from build123d import *

# Parameters (mm, degrees)
F1_DEPTH = 25
F2_W     = 113.5
F2_H     = 53.5
F3_DEPTH = 5
F5_DEPTH = 133.9
F6_W     = 113.5
F6_H     = 60
F7_DEPTH = 5
F9_DEPTH = 25


with BuildPart() as f1:
    # F0 (on Front) → F1 (new body)
    with BuildSketch(Plane.XZ):
        with BuildLine():
            Line((30.7684078276, 51.75), (-82.7315921724, 51.75))
            Line((-82.7315921724, 51.75), (-82.7315921724, 37.7107225358))
            Line((-82.7315921724, 37.7107225358), (-77.4815921724, 37.7107225358))
            ThreePointArc((-77.4815921724, 37.7107225358), (-73.9815921724, 41.2107225358), (-70.4815921724, 37.7107225358))
            Line((-70.4815921724, 37.7107225358), (-65.4815921724, 37.7107225358))
            ThreePointArc((-65.4815921724, 37.7107225358), (-61.9815921724, 41.2107225358), (-58.4815921724, 37.7107225358))
            Line((-58.4815921724, 37.7107225358), (-54.4815921724, 37.7107225358))
            ThreePointArc((-54.4815921724, 37.7107225358), (-50.9815921724, 41.2107225358), (-47.4815921724, 37.7107225358))
            Line((-47.4815921724, 37.7107225358), (-42.4815921724, 37.7107225358))
            ThreePointArc((-42.4815921724, 37.7107225358), (-38.9815921724, 41.2107225358), (-35.4815921724, 37.7107225358))
            Line((-35.4815921724, 37.7107225358), (-30.4815921724, 37.7107225358))
            ThreePointArc((-30.4815921724, 37.7107225358), (-26.9815921724, 41.2107225358), (-23.4815921724, 37.7107225358))
            Line((-23.4815921724, 37.7107225358), (-18.4815921724, 37.7107225358))
            ThreePointArc((-18.4815921724, 37.7107225358), (-14.9815921724, 41.2107225358), (-11.4815921724, 37.7107225358))
            Line((-11.4815921724, 37.7107225358), (-6.4815921724, 37.7107225358))
            ThreePointArc((-6.4815921724, 37.7107225358), (-2.9815921724, 41.2107225358), (0.5184078276, 37.7107225358))
            Line((0.5184078276, 37.7107225358), (5.5184078276, 37.7107225358))
            ThreePointArc((5.5184078276, 37.7107225358), (9.0184078276, 41.2107225358), (12.5184078276, 37.7107225358))
            Line((12.5184078276, 37.7107225358), (17.5184078276, 37.7107225358))
            ThreePointArc((17.5184078276, 37.7107225358), (21.0184078276, 41.2107225358), (24.5184078276, 37.7107225358))
            Line((24.5184078276, 37.7107225358), (30.7684078276, 37.7107225358))
            Line((30.7684078276, 37.7107225358), (30.7684078276, 51.75))
        make_face()
        with BuildLine():
            Line((-77.4815921724, 12.7484267578), (-82.7315921724, 12.7484267578))
            Line((-82.7315921724, 12.7484267578), (-82.7315921724, -1.75))
            Line((-82.7315921724, -1.75), (30.7684078276, -1.75))
            Line((30.7684078276, -1.75), (30.7684078276, 12.7484267578))
            Line((30.7684078276, 12.7484267578), (25.5184078276, 12.7484267578))
            ThreePointArc((25.5184078276, 12.7484267578), (22.0184078276, 9.2484267578), (18.5184078276, 12.7484267578))
            Line((18.5184078276, 12.7484267578), (13.5184078276, 12.7484267578))
            ThreePointArc((13.5184078276, 12.7484267578), (10.0184078276, 9.2484267578), (6.5184078276, 12.7484267578))
            Line((6.5184078276, 12.7484267578), (1.5184078276, 12.7484267578))
            ThreePointArc((1.5184078276, 12.7484267578), (-1.9815921724, 9.2484267578), (-5.4815921724, 12.7484267578))
            Line((-5.4815921724, 12.7484267578), (-10.4815921724, 12.7484267578))
            ThreePointArc((-10.4815921724, 12.7484267578), (-13.9815921724, 9.2484267578), (-17.4815921724, 12.7484267578))
            Line((-17.4815921724, 12.7484267578), (-22.4815921724, 12.7484267578))
            ThreePointArc((-22.4815921724, 12.7484267578), (-25.9815921724, 9.2484267578), (-29.4815921724, 12.7484267578))
            Line((-29.4815921724, 12.7484267578), (-34.4815921724, 12.7484267578))
            ThreePointArc((-34.4815921724, 12.7484267578), (-37.9815921724, 9.2484267578), (-41.4815921724, 12.7484267578))
            Line((-41.4815921724, 12.7484267578), (-46.4815921724, 12.7484267578))
            ThreePointArc((-46.4815921724, 12.7484267578), (-49.9815921724, 9.2484267578), (-53.4815921724, 12.7484267578))
            Line((-53.4815921724, 12.7484267578), (-58.4815921724, 12.7484267578))
            ThreePointArc((-58.4815921724, 12.7484267578), (-61.9815921724, 9.2484267578), (-65.4815921724, 12.7484267578))
            Line((-65.4815921724, 12.7484267578), (-70.4815921724, 12.7484267578))
            ThreePointArc((-70.4815921724, 12.7484267578), (-73.9815921724, 9.2484267578), (-77.4815921724, 12.7484267578))
        make_face()
        with BuildLine():
            Line((-77.4815921724, 37.7107225358), (-82.7315921724, 37.7107225358))
            Line((-82.7315921724, 37.7107225358), (-82.7315921724, 12.7484267578))
            Line((-82.7315921724, 12.7484267578), (-77.4815921724, 12.7484267578))
            ThreePointArc((-77.4815921724, 12.7484267578), (-73.9815921724, 16.2484267578), (-70.4815921724, 12.7484267578))
            Line((-70.4815921724, 12.7484267578), (-65.4815921724, 12.7484267578))
            ThreePointArc((-65.4815921724, 12.7484267578), (-61.9815921724, 16.2484267578), (-58.4815921724, 12.7484267578))
            Line((-58.4815921724, 12.7484267578), (-53.4815921724, 12.7484267578))
            ThreePointArc((-53.4815921724, 12.7484267578), (-49.9815921724, 16.2484267578), (-46.4815921724, 12.7484267578))
            Line((-46.4815921724, 12.7484267578), (-41.4815921724, 12.7484267578))
            ThreePointArc((-41.4815921724, 12.7484267578), (-37.9815921724, 16.2484267578), (-34.4815921724, 12.7484267578))
            Line((-34.4815921724, 12.7484267578), (-29.4815921724, 12.7484267578))
            ThreePointArc((-29.4815921724, 12.7484267578), (-25.9815921724, 16.2484267578), (-22.4815921724, 12.7484267578))
            Line((-22.4815921724, 12.7484267578), (-17.4815921724, 12.7484267578))
            ThreePointArc((-17.4815921724, 12.7484267578), (-13.9815921724, 16.2484267578), (-10.4815921724, 12.7484267578))
            Line((-10.4815921724, 12.7484267578), (-5.4815921724, 12.7484267578))
            ThreePointArc((-5.4815921724, 12.7484267578), (-1.9815921724, 16.2484267578), (1.5184078276, 12.7484267578))
            Line((1.5184078276, 12.7484267578), (6.5184078276, 12.7484267578))
            ThreePointArc((6.5184078276, 12.7484267578), (10.0184078276, 16.2484267578), (13.5184078276, 12.7484267578))
            Line((13.5184078276, 12.7484267578), (18.5184078276, 12.7484267578))
            ThreePointArc((18.5184078276, 12.7484267578), (22.0184078276, 16.2484267578), (25.5184078276, 12.7484267578))
            Line((25.5184078276, 12.7484267578), (30.7684078276, 12.7484267578))
            Line((30.7684078276, 12.7484267578), (30.7684078276, 37.7107225358))
            Line((30.7684078276, 37.7107225358), (24.5184078276, 37.7107225358))
            ThreePointArc((24.5184078276, 37.7107225358), (21.0184078276, 34.2107225358), (17.5184078276, 37.7107225358))
            Line((17.5184078276, 37.7107225358), (12.5184078276, 37.7107225358))
            ThreePointArc((12.5184078276, 37.7107225358), (9.0184078276, 34.2107225358), (5.5184078276, 37.7107225358))
            Line((5.5184078276, 37.7107225358), (0.5184078276, 37.7107225358))
            ThreePointArc((0.5184078276, 37.7107225358), (-2.9815921724, 34.2107225358), (-6.4815921724, 37.7107225358))
            Line((-6.4815921724, 37.7107225358), (-11.4815921724, 37.7107225358))
            ThreePointArc((-11.4815921724, 37.7107225358), (-14.9815921724, 34.2107225358), (-18.4815921724, 37.7107225358))
            Line((-18.4815921724, 37.7107225358), (-23.4815921724, 37.7107225358))
            ThreePointArc((-23.4815921724, 37.7107225358), (-26.9815921724, 34.2107225358), (-30.4815921724, 37.7107225358))
            Line((-30.4815921724, 37.7107225358), (-35.4815921724, 37.7107225358))
            ThreePointArc((-35.4815921724, 37.7107225358), (-38.9815921724, 34.2107225358), (-42.4815921724, 37.7107225358))
            Line((-42.4815921724, 37.7107225358), (-47.4815921724, 37.7107225358))
            ThreePointArc((-47.4815921724, 37.7107225358), (-50.9815921724, 34.2107225358), (-54.4815921724, 37.7107225358))
            Line((-54.4815921724, 37.7107225358), (-58.4815921724, 37.7107225358))
            ThreePointArc((-58.4815921724, 37.7107225358), (-61.9815921724, 34.2107225358), (-65.4815921724, 37.7107225358))
            Line((-65.4815921724, 37.7107225358), (-70.4815921724, 37.7107225358))
            ThreePointArc((-70.4815921724, 37.7107225358), (-73.9815921724, 34.2107225358), (-77.4815921724, 37.7107225358))
        make_face()
    extrude(amount=F1_DEPTH)

    # F2 (on face) → F3 (join)
    with BuildSketch(Plane(origin=(0, 0, 0), x_dir=(-1, 0, 0), z_dir=(0, 1, 0))):
        with Locations((25.9815921724, 25)):
            Rectangle(F2_W, F2_H)
    extrude(amount=F3_DEPTH)

    # F4 (on face) → F5 (cut)
    with BuildSketch(Plane(origin=(-82.7315921724, 0, 0), x_dir=(0, -1, 0), z_dir=(-1, 0, 0))):
        Polygon((25, -1.75), (25, 51.75), (16.1387622356, -1.75), align=None)
    extrude(amount=-F5_DEPTH, mode=Mode.SUBTRACT)

    # F6 (on face) → F7 (join)
    with BuildSketch(Plane.XY.offset(51.75)):
        with Locations((-25.9815921724, -25)):
            Rectangle(F6_W, F6_H)
    extrude(amount=F7_DEPTH)

    # F8 (on face) → F9 (cut)
    with BuildSketch(Plane(origin=(0, 0, 51.75), x_dir=(1, 0, 0), z_dir=(0, 0, -1))):
        with BuildLine():
            ThreePointArc((-63.7315921724, 45), (-65.9815921724, 47.25), (-68.2315921724, 45))
            Line((-68.2315921724, 45), (-63.7315921724, 45))
        make_face()
        with BuildLine():
            ThreePointArc((16.2684078276, 45), (14.0184078276, 47.25), (11.7684078276, 45))
            Line((11.7684078276, 45), (16.2684078276, 45))
        make_face()
        with BuildLine():
            Line((16.2684078276, 45), (11.7684078276, 45))
            ThreePointArc((11.7684078276, 45), (14.0184078276, 42.75), (16.2684078276, 45))
        make_face()
        with BuildLine():
            ThreePointArc((-23.7315921724, 45), (-25.9815921724, 47.25), (-28.2315921724, 45))
            Line((-28.2315921724, 45), (-23.7315921724, 45))
        make_face()
        with BuildLine():
            Line((-23.7315921724, 45), (-28.2315921724, 45))
            ThreePointArc((-28.2315921724, 45), (-25.9815921724, 42.75), (-23.7315921724, 45))
        make_face()
        with BuildLine():
            Line((-63.7315921724, 45), (-68.2315921724, 45))
            ThreePointArc((-68.2315921724, 45), (-65.9815921724, 42.75), (-63.7315921724, 45))
        make_face()
        with BuildLine():
            ThreePointArc((-63.7315921724, 35), (-65.9815921724, 37.25), (-68.2315921724, 35))
            Line((-68.2315921724, 35), (-63.7315921724, 35))
        make_face()
        with BuildLine():
            ThreePointArc((16.2684078276, 35), (14.0184078276, 37.25), (11.7684078276, 35))
            Line((11.7684078276, 35), (16.2684078276, 35))
        make_face()
        with BuildLine():
            Line((16.2684078276, 35), (11.7684078276, 35))
            ThreePointArc((11.7684078276, 35), (14.0184078276, 32.75), (16.2684078276, 35))
        make_face()
        with BuildLine():
            ThreePointArc((-23.7315921724, 35), (-25.9815921724, 37.25), (-28.2315921724, 35))
            Line((-28.2315921724, 35), (-23.7315921724, 35))
        make_face()
        with BuildLine():
            Line((-23.7315921724, 35), (-28.2315921724, 35))
            ThreePointArc((-28.2315921724, 35), (-25.9815921724, 32.75), (-23.7315921724, 35))
        make_face()
        with BuildLine():
            Line((-63.7315921724, 35), (-68.2315921724, 35))
            ThreePointArc((-68.2315921724, 35), (-65.9815921724, 32.75), (-63.7315921724, 35))
        make_face()
    extrude(amount=-F9_DEPTH, mode=Mode.SUBTRACT)


solid = f1.part
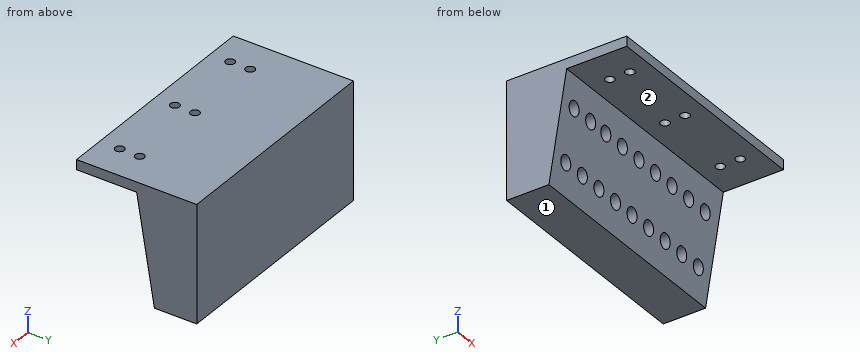
Source: CAD feature listing. Evaluate the final solid. Frame: model axes, mm. Face numbers are marked on the shaded views. A direction names the side the tool comes from. Give positions to 0.01 mm unless a question says otherwise; leave off trailing zeros. Order: outer loops, then holes, each group sorted by start corner. A loop starts at its lowest first (then second) coordinate and runs counter-clockwise, first axis right, second up. Notation, with made-up numbers: (46.25, 45) -> (81.25, 45) arc R20 cw to (81.25, 50) -> close; hole circle Ø8 at (-11.75, 57). An arc over 180 degrees is marked (long way). Use a Markdown table: item, result.
1) Section query B-B, the plane x = -32.5. Return the cut outline in (y, z), then the cut area to 3 significant figures.
Answer list:
| item | result |
|---|---|
| outline | (-55, 51.75) -> (-25, 51.75) -> (-16.14, -1.75) -> (5, -1.75) -> (5, 56.75) -> (-55, 56.75) -> close |
| area | 1,670 mm² |
2) Section query C-C, the plane y = -21. Count the separate pieces of the cut face and the enclosed holes in it, then the cut area to 3 significant figures.
Answer list:
| item | result |
|---|---|
| separate pieces | 1 |
| enclosed holes | 9 |
| area | 2,960 mm² |
3) Contact query for flat-ended pins moving along their axis: P1, Ø3, axis at x = -55, y = -38.5, coming from the -Z side; P2, Ø6.5, axis at x = -13.98, z = 12.75, coming from the -Y side; P3, Ø5, axis at x = -46.5, z = 20, coming from the -Y side. Output: stop coordinate, or through.
Answer list:
| item | result |
|---|---|
| P1 | z = 51.75 |
| P2 | y = 0 |
| P3 | y = -20.16 |
4) Section query A-A, the plane y = -45. Return the cut outline in (x, z), then the cut area to 3 significant figures.
Answer list:
| item | result |
|---|---|
| outline | (-82.73, 51.75) -> (-68.23, 51.75) -> (-68.23, 56.75) -> (-82.73, 56.75) -> close; (-63.73, 51.75) -> (-28.23, 51.75) -> (-28.23, 56.75) -> (-63.73, 56.75) -> close; (-23.73, 51.75) -> (11.77, 51.75) -> (11.77, 56.75) -> (-23.73, 56.75) -> close; (16.27, 51.75) -> (30.77, 51.75) -> (30.77, 56.75) -> (16.27, 56.75) -> close |
| area | 500 mm² |
5) Ray query, line 1 along Z through (x, y) = (-28, -15.5); line 2 along Z through (x, y) = (10.5, -16); line 3 along Z through (x, y) = (-62.5, -31). Return the intervals inside material, ascending. Write a range as [from, to].
Answer list:
| item | result |
|---|---|
| line 1 | [-1.75, 9.89], [15.61, 34.36], [41.06, 56.75] |
| line 2 | [-1.75, 9.28], [16.22, 34.54], [40.88, 56.75] |
| line 3 | [51.75, 56.75] |
6) Reachability of the marked faces 1 and 2 from +Z, -Z, +X, -X, +Y, -Y: full face, straight path, thin tool, end or side. Return the list, or none.
Answer list:
| item | result |
|---|---|
| face 1 | -Z, +X, -X, +Y, -Y |
| face 2 | -Z, +X, -X, -Y |
